Could you check a few things on this model? Use its own coordinates, in mm. A direction names the side the tool comes from. Round coordinates to 2 decimals unless told otherwise and drop trailing zeros. Order: outer loops, then holes, each group sorted by start corner. A loop starts at its lowest first (then second) coordinate and runs counter-clockwise, first axis right, second up.
```python
from build123d import *

# Parameters (mm, degrees)
SKETCH1_R           = 36
SKETCH1_R_2         = 32
BOSS_EXTRUDE1_DEPTH = 10
CIRPATTERN1_COUNT   = 2
CIRPATTERN1_ANGLE   = 16
CIRPATTERN2_COUNT   = 2


with BuildPart() as part:
    # Sketch1 → Boss-Extrude1 (new, symmetric)
    with BuildSketch(Plane.XY):
        Circle(SKETCH1_R)
        Circle(SKETCH1_R_2, mode=Mode.SUBTRACT)
    extrude(amount=BOSS_EXTRUDE1_DEPTH, both=True)

    # Sketch5 → Revolve1 (revolve)
    with BuildSketch(Plane(origin=(0, 0, 0), x_dir=(0, 0, -1), z_dir=(1, 0, 0))):
        Polygon((6, 32), (6, 38.5), (6.5, 38.5), (6.5, 44.5), (8, 44.5), (8, 32), align=None)
    revolve1 = revolve(axis=Axis((0, 44.5, -8), (0, -1, 0)))

    # CirPattern1: Revolve1 ×2 about axis
    cirpattern1_axis = Axis((0, 0, 10), (0, 0, 1))
    for i in range(1, CIRPATTERN1_COUNT):
        add(revolve1.rotate(cirpattern1_axis, i * CIRPATTERN1_ANGLE / (CIRPATTERN1_COUNT - 1)))

    # CirPattern2: Revolve1 ×2 about axis
    cirpattern2_axis = Axis((0, 0, 10), (0, 0, -1))
    for i in range(1, CIRPATTERN2_COUNT):
        add(revolve1.rotate(cirpattern2_axis, i * 360 / CIRPATTERN2_COUNT))

    # CirPattern2 copy 1 sketch → CirPattern2 copy 1 (revolve)
    with BuildSketch(Plane(origin=(0, 0, 0), x_dir=(0, 0, -1), z_dir=(-0.9612616959383187, -0.2756373558169999, 0))):
        Polygon((6, 32), (6, 38.5), (6.5, 38.5), (6.5, 44.5), (8, 44.5), (8, 32), align=None)
    revolve(axis=Axis((12.265862334, -42.776145469, -8), (-0.2756373558169999, 0.9612616959383187, 0)))


solid = part.part
```
Q1. I need wall thicknesses on L1, parallel to Y at x = 0, z = 0.25; L2, parallel to Y at x = -27.5, z = 2.75. Which ranges of each line are inside material? Lowest first, please.
Q2. For P1, Ø1.5, axis at y = -6, z = -5, coming from the +X side; P2, Ø8, axis at y = -28, z = 7, coming from the -X side; P3, Ø6, axis at y = -26, z = 3, coming from the -X side, each with a flat end and sliding along its axis, tell me the tip position at first contact or that it passes through.
Q3. Imagine slicing it at B-B, the plane x = -21.5. Please give me the cut outline in (y, z), then the cut area to 3 significant figures.
Q4. Imagine slicing it at A-A, the plane y = 0. Please give me the cut outline in (x, z), then the cut area to 3 significant figures.
Q5. We'd pull the mould along Y, two halves only. Please class faces 4 (the flat face through (-12.29, 42.77, -8.02)), 5 (the cylindrical face through (0.07, -41.54, -9.5)), 6 (the cylindrical face through (-6.94, -31.24, -0.14)): released by +Y, released by -Y, zero draft, split by the parting line, or undercut.
Q6. Imagine slicing it at C-C, the plane z = -4.5. Please give me the cut outline in (x, y).
Q7. For faces 1 (the cylindrical face through (1.2, 37.2, -9.6)), 2 (the cylindrical face through (0, -37, -10)), 3 (the flat face through (0, 44.5, -8)), which set-ups out of +Z, -Z, +X, -X, +Y, -Y let a thin tool reach every point of the face, with its end or its side?
Filled in:
1. L1: y = -36 to -32, 32 to 36
1. L2: y = -23.23 to -16.36, 16.36 to 23.23
2. P1: stops at x = 35.62
2. P2: stops at x = -26.83
2. P3: stops at x = -27.69
3. outline: (-28.87, -10) - (-23.7, -10) - (-23.7, 10) - (-28.87, 10) - close; (23.7, -10) - (28.87, -10) - (28.87, 10) - (23.7, 10) - close
3. area: 207 mm2
4. outline: (-36, -10) - (-32, -10) - (-32, 10) - (-36, 10) - close; (32, -10) - (36, -10) - (36, 10) - (32, 10) - close
4. area: 160 mm2
5. face 4: released by +Y
5. face 5: zero draft
5. face 6: undercut
6. outline: circle Ø72 at (0, 0); hole circle Ø64 at (0, 0)
7. face 1: +Y
7. face 2: -Y
7. face 3: +Z, -Z, +X, -X, +Y
